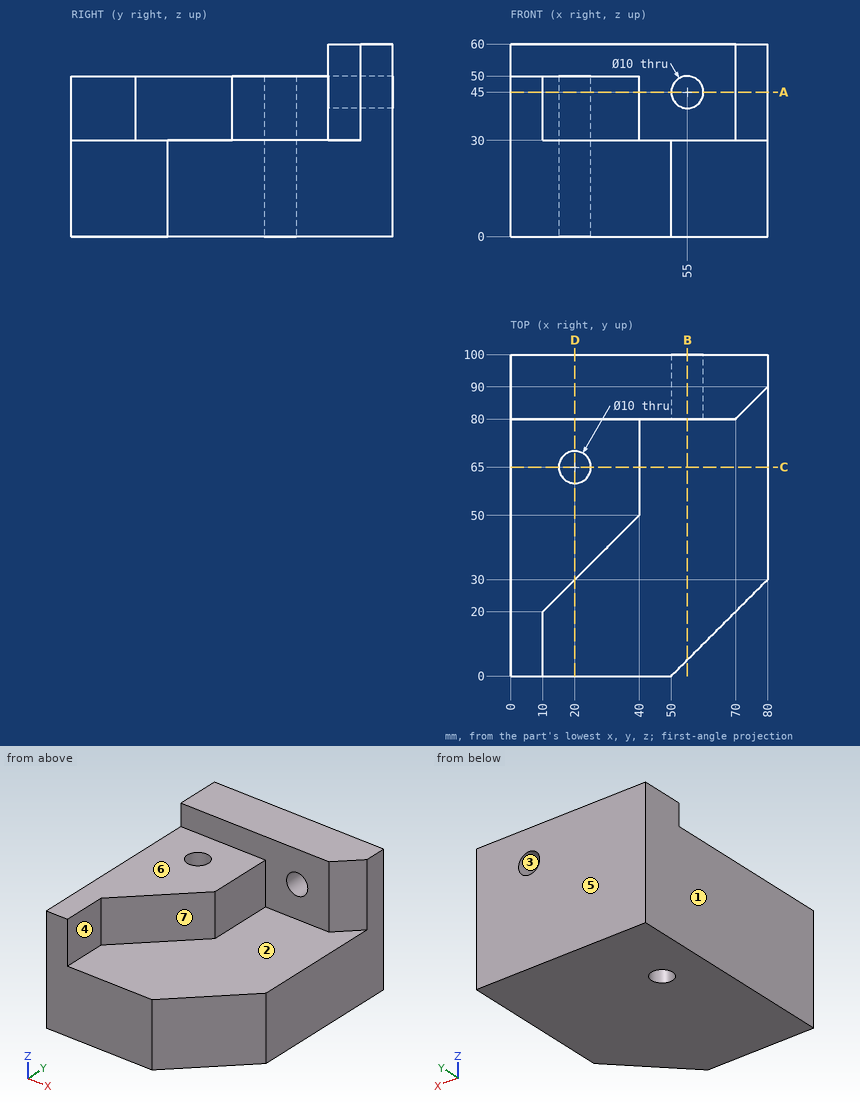
Part print with two shaded views. Sizes in mm from the minimum x, y, z corner. A direction names the side the tool comes from. Round coordinates to 2 decimals unless told otherwise and drop trailing zeros. Order: outer loops, then holes, each group sorted by start corner. A loop starts at its lowest first (then second) coordinate and runs counter-clockwise, first axis right, second up. Notation, with made-up numbers: M 38.25,20 L 74.25,20 A17 cw 74.25,24 Z; hole C 53.5,-10.75 d10. An arc over 180 degrees is marked long. Put each result on its own line as item: value. Start each with the question number.
1. Drill centre lines: probe 1 along Z at (x, y) = (34, 31); probe 2 along Y at (x, z) = (20, 32); probe 3 along Y at (x, z) = (20, 26). Where is each one in solid material? Low to high. Write a range as [from, to].
2. Drop flat-ended pins along their axis: pin 1 (1 mm diameter, centred on y = 40.5, z = 32, fed in from -X); pin 2 (1.5 mm diameter, centred on y = 20.5, z = 44.5, fed in from +X); pin 3 (4 mm diameter, centred on x = 30, z = 43.5, fed in from -Y); pin 4 (10 mm diameter, centred on y = 59.5, z = 42, fed in from +X). Give the stop position or say it passes through.
3. Slice it at D-D on x = 20. List the corners of the cut face in (y, z).
4. Two-plate mould, pull along X, no slides. Class the marked faces 1, 2, 3 and 4: +X half, -X half, draft (parallel to the pull), parting line (faces both ways), or undercut.
5. Slice it at A-A on z = 45. List the corners of the cut face in (x, y).
6. Slice it at C-C on y = 65. List the corners of the cut face in (x, z), then the cut area to 3 significant figures.
7. Tool access for the marked faces 5, 6 and 7: list every direction of +Z, -Z, +X, -X, +Y, -Y with a clear straight run to the whole face (end or side of a thin tool).
8. Slice it at B-B on x = 55. List the corners of the cut face in (y, z), then the cut area to 3 significant figures.
Findings:
1. probe 1: [0, 30]
1. probe 2: [30, 60], [70, 100]
1. probe 3: [0, 60], [70, 100]
2. pin 1: x = 0
2. pin 2: x = 11.25
2. pin 3: y = 38
2. pin 4: x = 40
3. outline: M 0,0 L 60,0 L 60,50 L 30,50 L 30,30 L 0,30 Z; M 70,0 L 100,0 L 100,60 L 80,60 L 80,50 L 70,50 Z
4. face 1: -X half
4. face 2: draft
4. face 3: undercut
4. face 4: +X half
5. outline: M 0,0 L 10,0 L 10,20 L 40,50 L 40,80 L 50,80 L 50,100 L 0,100 Z; M 60,80 L 70,80 L 80,90 L 80,100 L 60,100 Z; hole C 20,65 d10
6. outline: M 0,0 L 15,0 L 15,50 L 0,50 Z; M 25,0 L 80,0 L 80,30 L 40,30 L 40,50 L 25,50 Z
6. area: 2,700 mm2
7. face 5: +Z, -Z, +X, -X, +Y
7. face 6: +Z, +X, -X, -Y
7. face 7: +Z, +X, -Y
8. outline: M 5,0 L 100,0 L 100,40 L 80,40 L 80,30 L 5,30 Z; M 80,50 L 100,50 L 100,60 L 80,60 Z
8. area: 3,250 mm2
